Design review of the part built by this model. Coordinates are the model's own, in mm. A direction names the side the tool comes from. Give positions to 0.01 mm unless a question says otherwise; leave off trailing zeros. Loops run counter-clockwise (first coordinate to the right, second up) from the corner with the lowest first, then second, coordinate; pieces in that order, holes last. Notation, with made-up numbers: M 77.5,44.25 L 121.5,44.25 A25 ccw 121.5,59.25 Z; hole C 86,68.25 d9. An arc over 180 degrees is marked long. Use one line per item in the form item = value. Start each with the question number.
from build123d import *

# Parameters (mm, degrees)
BOSS_EXTRU_1_DEPTH  = 4
SKETCH1_R           = 3.25
SKETCH1_R_2         = 2.25
BOSS_EXTRUDE1_DEPTH = 2
SKETCH1_3_R         = 2.75
SKETCH1_3_R_2       = 1.5
BOSS_EXTRUDE2_DEPTH = 1


with BuildPart() as part:
    # Esquisse1 → Boss.-Extru.1 (new body)
    with BuildSketch(Plane.XY):
        with BuildLine():
            Line((-2.61937647, 2.683536269), (-2.736999418, 0.267084608))
            ThreePointArc((-2.736999418, 0.267084608), (-0.026847744, 2.749868942), (2.731262929, 0.320472792))
            Line((2.731262929, 0.320472792), (2.591528882, 2.71043872))
            ThreePointArc((2.591528882, 2.71043872), (-0.019359946, 3.749950025), (-2.61937647, 2.683536269))
        make_face()
        with BuildLine():
            ThreePointArc((2.731262929, 0.320472792), (2.745311736, 0.160510037), (2.75, 0))
            ThreePointArc((2.75, 0), (2.745311736, -0.160510037), (2.731262929, -0.320472792))
            Line((2.731262929, -0.320472792), (2.591528882, -2.71043872))
            ThreePointArc((2.591528882, -2.71043872), (3.448241096, -1.473815913), (3.75, 0))
            ThreePointArc((3.75, 0), (3.448241096, 1.473815913), (2.591528882, 2.71043872))
            Line((2.591528882, 2.71043872), (2.731262929, 0.320472792))
        make_face()
        with BuildLine():
            ThreePointArc((2.731262929, -0.320472792), (-0.026847744, -2.749868942), (-2.736999418, -0.267084608))
            Line((-2.736999418, -0.267084608), (-2.61937647, -2.683536269))
            ThreePointArc((-2.61937647, -2.683536269), (-0.019359946, -3.749950025), (2.591528882, -2.71043872))
            Line((2.591528882, -2.71043872), (2.731262929, -0.320472792))
        make_face()
        with BuildLine():
            ThreePointArc((-2.736999418, -0.267084608), (-2.746747932, -0.133700414), (-2.75, 0))
            ThreePointArc((-2.75, 0), (-2.746747932, 0.133700414), (-2.736999418, 0.267084608))
            Line((-2.736999418, 0.267084608), (-2.61937647, 2.683536269))
            ThreePointArc((-2.61937647, 2.683536269), (-3.75, 0), (-2.61937647, -2.683536269))
            Line((-2.61937647, -2.683536269), (-2.736999418, -0.267084608))
        make_face()
    extrude(amount=BOSS_EXTRU_1_DEPTH)

    # Sketch1 → Boss-Extrude1 (add)
    # profile 1 of 2: a face of its own
    with BuildSketch(Plane(origin=(0, 0, 0), x_dir=(-1, 0, 0), z_dir=(0, 0, -1))):
        with BuildLine():
            ThreePointArc((3.25, 30), (0, 26.75), (-3.25, 30))
            Line((-3.25, 30), (-3.747917245, 0.124965287))
            ThreePointArc((-3.747917245, 0.124965287), (0, 3.75), (3.747917245, 0.124965287))
            Line((3.747917245, 0.124965287), (3.25, 30))
        make_face()
    # profile 2 of 2: a face of its own
    with BuildSketch(Plane(origin=(0, 0, 0), x_dir=(-1, 0, 0), z_dir=(0, 0, -1))):
        with Locations((0, 30)):
            Circle(SKETCH1_R)
        with Locations((0, 30)):
            Circle(SKETCH1_R_2, mode=Mode.SUBTRACT)
    extrude(amount=-BOSS_EXTRUDE1_DEPTH)

    # Sketch1_3 → Boss-Extrude2 (add)
    with BuildSketch(Plane(origin=(0, 0, 0), x_dir=(-1, 0, 0), z_dir=(0, 0, -1))):
        Circle(SKETCH1_3_R)
        Circle(SKETCH1_3_R_2, mode=Mode.SUBTRACT)
    extrude(amount=-BOSS_EXTRUDE2_DEPTH)


solid = part.part
Q1. Wall thickness on probe 1 along Y at (x, z) = (0, 0.75); probe 2 along Y at (x, z) = (-1.25, 1.85); probe 3 along Z at (x, y) = (-2.5, 29): over which ranges is each line inside the solid? List them lowest first.
Q2. The part is to be moulded in two halves that separate along Y. For faces 3 (the flat face through (0, 17, 2)), 4 (the cylindrical face through (1.5, 0.07, 0.49)), 5 (the cylindrical face through (-0.07, 33.25, 0.99)), say which applies: pulls with the +Y half, pulls with the -Y half, needs draft (parallel to the pull), parting line crosses it, or undercut.
Q3. Take a section at D-D on y = 13.5. Give the boundary of the cut face in (x, z) (3 decimals), plus the area to 3 significant figures.
Q4. Take a section at C-C on y = 29.5. Give the boundary of the cut face in (x, z), plus the area to 3 significant figures.
Q5. Take a section at B-B on x = 0. Give the boundary of the cut face in (y, z).
Q6. For faces 1 (the flat face through (-1.2, -1.2, 1)), 2 (the flat face through (0, 15, 0)), list the 3-axis set-ups (+Z, -Z, +X, -X, +Y, -Y) from which the entire face can be reached by the end or side of a thin tool; tool diameter is ignored.
Q7. Clearance check with flat-ended pins moving along their axes: pin 1 Ø4 at (x, y) = (0, 30) entering from -Z; pin 2 Ø1 at (x, y) = (2.5, 14) entering from +Z. State where each tip first meets the part, or that it passes through.
Q8. Take a section at A-A on z = 3.3. Give the boundary of the cut face in (x, y).
Response values:
q1.probe_1 = -3.75 to -1.5, 1.5 to 27.75, 32.25 to 33.25
q1.probe_2 = -3.54 to -2.45, 2.45 to 28.13, 31.87 to 33
q1.probe_3 = 0 to 2
q2.face_3 = needs draft
q2.face_4 = undercut
q2.face_5 = pulls with the +Y half
q3.outline = M -3.525,0 L 3.525,0 L 3.525,2 L -3.525,2 Z
q3.area = 14.1 mm^2
q4.outline = M -3.26,0 L -2.19,0 L -2.19,2 L -3.26,2 Z; M 2.19,0 L 3.26,0 L 3.26,2 L 2.19,2 Z
q4.area = 4.26 mm^2
q5.outline = M -3.75,0 L -1.5,0 L -1.5,1 L -2.75,1 L -2.75,4 L -3.75,4 Z; M 1.5,0 L 27.75,0 L 27.75,2 L 3.75,2 L 3.75,4 L 2.75,4 L 2.75,1 L 1.5,1 Z; M 32.25,0 L 33.25,0 L 33.25,2 L 32.25,2 Z
q6.face_1 = +Z
q6.face_2 = -Z, +X, -X, +Y, -Y
q7.pin_1 = through
q7.pin_2 = 2
q8.outline = C 0,0 d7.5; hole C 0,0 d5.5
